Study the drawing (mm; zero at the part's minimum x, y, z) and answer. Give positions to 0.01 mm unless a question says otherwise; leave off trailing zeros. Order: outer loops, then holes, each group sorted by start corner. A loop starts at its lowest first (then second) coordinate and runs counter-clockwise, first axis right, second up. Notation, with made-up numbers: (81, 12.25) - (110, 12.25) arc R34 cw to (110, 47.25) - close; hole circle Ø3 at (17, -26). An arc over 180 degrees is marked (long way). Return JSON: item names as keys, results as strings.
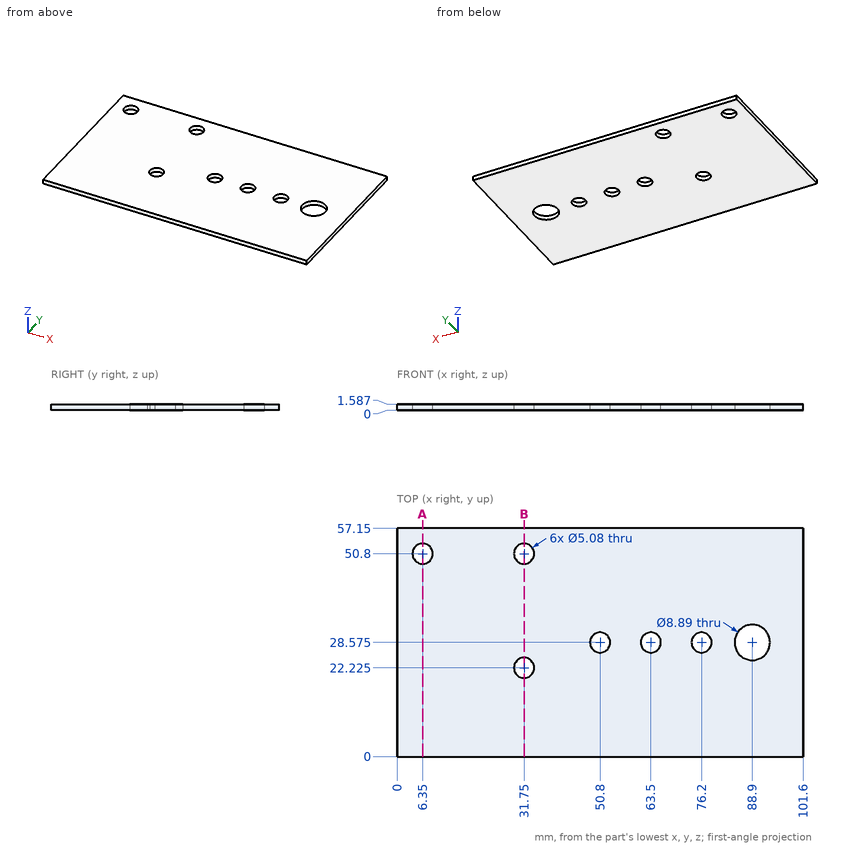
Q1. A cutting plane is placed at A-A (x = 6.35). Write down the section's boundary in (y, z).
Values:
{"outline": "(0, 0) - (48.26, 0) - (48.26, 1.59) - (0, 1.59) - close; (53.34, 0) - (57.15, 0) - (57.15, 1.59) - (53.34, 1.59) - close"}
Q2. Given pin 1 (8 mm diameter, centred on x = 88.9, y = 28.575, fed in from +Z), flat-ended and moving along its own axis, determine where the tip first touches the part or whether it passes through.
Values:
{"pin 1": "passes through"}
Q3. Consider L1, parallel to Y at x = 6.35, z = 1.15; L2, parallel to X at y = 29, z = 0.5 (1 decimal); L3, parallel to Y at x = 76.5, z = 1.1. Determine where each line is inside the solid, lowest interval first.
Values:
{"L1": "y = 0 to 48.26, 53.34 to 57.15", "L2": "x = 0 to 48.3, 53.3 to 61, 66 to 73.7, 78.7 to 84.5, 93.3 to 101.6", "L3": "y = 0 to 26.05, 31.1 to 57.15"}
Q4. A cutting plane is placed at B-B (x = 31.75). Give the number of separate pieces and of enclosed holes in the cut face.
Values:
{"separate pieces": "3", "enclosed holes": "0"}
